```python
from build123d import *

# Parameters (mm, degrees)
F0_R     = 19.05
F0_R_2   = 15.24
F1_DEPTH = 50.8
F3_DEPTH = 25.4
F4_W     = 30.48
F4_H     = 30.48
F5_DEPTH = 25.4


with BuildPart() as f1:
    # F0 (on Top) → F1 (new body)
    with BuildSketch(Plane.XY):
        Circle(F0_R)
        Circle(F0_R_2, mode=Mode.SUBTRACT)
    extrude(amount=F1_DEPTH)

    # F2 (on Front) → F3 (cut, symmetric)
    with BuildSketch(Plane.XZ):
        Polygon((19.165186, 50.845042), (-19.072151, 50.938074), (19.165186, 38.006227), align=None)
    extrude(amount=F3_DEPTH, both=True, mode=Mode.SUBTRACT)

    # F4 (on Right) → F5 (cut)
    with BuildSketch(Plane.YZ):
        with Locations((-0.046517, 29.21)):
            Rectangle(F4_W, F4_H)
    extrude(amount=F5_DEPTH, mode=Mode.SUBTRACT)


solid = f1.part
```
Here's how the part is built. I have some questions about the finished solid (model axes, mm). A direction names the side the tool comes from. Coordinates: 2 decimals unless noted, no trailing zeros. Loops run counter-clockwise (first coordinate to the right, second up) from the corner with the lowest first, then second, coordinate; pieces in that order, holes last. Notation, with made-up numbers: (12.25, 78) - (30.25, 78) arc R32 ccw to (30.25, 106) - close; hole circle Ø7 at (7.25, 5.5). An arc over 180 degrees is marked (long way). Answer as CSV lines item,"result".
Q1. For faces 5 (the face through (16, 1, 13.97)), 6 (the face through (-9, 13, 0)), which set-ups out of +Z, -Z, +X, -X, +Y, -Y let a thin tool reach every point of the face, with its end or its side?
Response:
face 5,"+Z, +X"
face 6,"-Z, +X, -X, +Y, -Y"
Q2. If we section it at D-D, the plane z = 38: Write out the boundary of the cut face in (x, y), and give its area (3 significant figures).
Response:
outline,"(0, -15.29) - (0, -15.24) arc R15.24 cw (long way) to (1.19, 15.19) - (11.49, 15.19) arc R19.05 ccw (long way) to (11.37, -15.29) - close"
area,"265 mm2"
Q3. If we section it at A-A, the plane y = 0: Write out the boundary of the cut face in (x, z).
Response:
outline,"(-19.05, 0) - (-15.24, 0) - (-15.24, 49.64) - (-18.66, 50.8) - (-19.05, 50.8) - close; (15.24, 0) - (19.05, 0) - (19.05, 13.97) - (15.24, 13.97) - close"
Q4. We'd pull the mould along Y, two halves only. Please class faces 1 (the face through (6, 15.193, 29)), 2 (the face through (-19.03, 0.84, 19.4)), 3 (the face through (-15.225, 0.67, 19.039)), 4 (the face through (-14.825, -4.322, 49.502)): pulls with the +Y half, pulls with the -Y half, needs draft (parallel to the pull), parting line crosses it, or undercut.
Response:
face 1,"undercut"
face 2,"parting line crosses it"
face 3,"undercut"
face 4,"needs draft"
Q5. If we section it at B-B, the plane z = 4: Write out the boundary of the cut face in (x, y).
Response:
outline,"circle Ø38.1 at (0, 0); hole circle Ø30.48 at (0, 0)"
Q6. For pin 1 (1 mm diameter, centred on x = -5.5, z = 41.5, fed in from -Y); pin 2 (5 mm diameter, centred on x = -9.5, y = 8, fed in from -Z); pin 3 (21 mm diameter, centred on x = 5.5, y = -2.5, fed in from +Z); pin 4 (1 mm diameter, centred on y = -11.5, z = 10, fed in from -X), each with a flat end and sliding along its axis, tell me the tip position at first contact or that it passes through.
Response:
pin 1,"y = -18.38"
pin 2,"through"
pin 3,"z = 13.97"
pin 4,"x = -15.55"
Q7. If we section it at C-C, the plane x = -6: Write out the boundary of the cut face in (y, z), and give its area (3 significant figures).
Response:
outline,"(-18.08, 0) - (-14.01, 0) - (-14.01, 46.52) - (-18.08, 46.52) - close; (14.01, 0) - (18.08, 0) - (18.08, 46.52) - (14.01, 46.52) - close"
area,"379 mm2"
Q8. If I drill on L1, parallel to Y at x = 0, z = 13.5; L2, parallel to Y at x = 0, z = 25; L3, parallel to Z at x = 3, y = 15, over which ranges is the centre line in solid material (lowest first)? Write a range as [from, to].
Response:
L1,"[-19.05, -15.24], [15.24, 19.05]"
L2,"[-19.05, -15.29], [15.24, 19.05]"
L3,"[0, 13.97]"
